Input: part model. Units: mm. Frame: model coordinates. Face numbers are marked on the shaded views. Coordinates: 2 decimals unless noted, no trailing zeros. Order: outer loops, then holes, each group sorted by start corner. A loop starts at its lowest first (then second) coordinate and runs counter-clockwise, first axis right, second up. Notation, with made-up numbers: (77.25, -0.75) - (116.25, -0.75) arc R23 cw to (116.25, 26.25) - close; hole circle Ø1 at (-2, 12.25). An arc over 180 degrees is marked (long way). One line per question, with ' | ' between items.
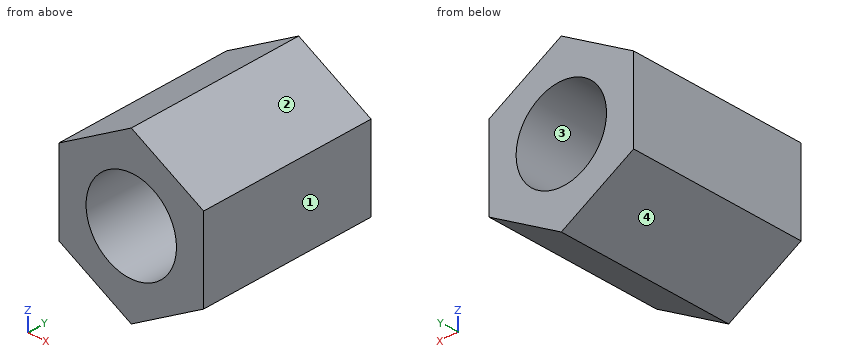
from build123d import *

# Parameters (mm, degrees)
SKETCH_R  = 1.75
PAD_DEPTH = 7


with BuildPart() as part:
    # Sketch → Pad (new body)
    with BuildSketch(Plane.XZ):
        Polygon((2.8, 1.616581), (0, 3.233162), (-2.8, 1.616581), (-2.8, -1.616581), (0, -3.233162), (2.8, -1.616581), align=None)
        Circle(SKETCH_R, mode=Mode.SUBTRACT)
    extrude(amount=PAD_DEPTH)


solid = part.part
Item 1: Draft query along Z for the marked faces 1, 2, 3 and 4. Return one class per face: released by +Z, released by -Z, zero draft, split by the parting line, or undercut.
Data:
face 1: zero draft | face 2: released by +Z | face 3: undercut | face 4: released by -Z
Item 2: Section A-A on z = 0. Return the cut outline in (x, y), and give its area (3 significant figures).
Data:
outline: (-2.8, -7) - (-1.75, -7) - (-1.75, 0) - (-2.8, 0) - close; (1.75, -7) - (2.8, -7) - (2.8, 0) - (1.75, 0) - close | area: 14.7 mm^2
Item 3: Section C-C on x = 1.15. Return the cut outline in (y, z), and give its area (3 significant figures).
Data:
outline: (-7, -2.57) - (0, -2.57) - (0, -1.32) - (-7, -1.32) - close; (-7, 1.32) - (0, 1.32) - (0, 2.57) - (-7, 2.57) - close | area: 17.5 mm^2
Item 4: Ray query, line 1 (Z direction, x = 1.5, y = -6.5); line 2 (Z direction, x = -1.3, y = -5.5); line 3 (X direction, y = -6.5, z = -1.5). Return the intervals inside material, ascending.
Data:
line 1: -2.37 to -0.9, 0.9 to 2.37 | line 2: -2.48 to -1.17, 1.17 to 2.48 | line 3: -2.8 to -0.9, 0.9 to 2.8
Item 5: Section B-B on y = -1. Return the cut outline in (x, z).
Data:
outline: (-2.8, -1.62) - (0, -3.23) - (2.8, -1.62) - (2.8, 1.62) - (0, 3.23) - (-2.8, 1.62) - close; hole circle Ø3.5 at (0, 0)
Item 6: Section D-D on z = -2. Return the cut outline in (x, y).
Data:
outline: (-2.14, -7) - (2.14, -7) - (2.14, 0) - (-2.14, 0) - close
